from build123d import *

# Parameters (mm, degrees)
BOSS_EXTRUDE1_DEPTH = 25.4
SKETCH2_R           = 2.159
CUT_EXTRUDE1_DEPTH  = 25.4
SKETCH3_R           = 2.159
CUT_EXTRUDE2_DEPTH  = 25.4


with BuildPart() as part:
    # Sketch1 → Boss-Extrude1 (new body)
    with BuildSketch(Plane.XY):
        Polygon((-9.009241013, -10.149737798), (-28.059241013, -10.149737798), (-28.059241013, -6.974737798), (-12.819241013, -6.974737798), (-12.819241013, 5.598262202), (6.738758987, 5.598262202), (6.738758987, -6.974737798), (21.978758987, -6.974737798), (21.978758987, -10.149737798), (2.928758987, -10.149737798), (2.928758987, 1.788262202), (-9.009241013, 1.788262202), align=None)
    extrude(amount=BOSS_EXTRUDE1_DEPTH)

    # Sketch2 → Cut-Extrude1 (cut)
    with BuildSketch(Plane(origin=(0, -6.974737798, 0), x_dir=(1, 0, 0), z_dir=(0, 1, 0))):
        with Locations((14.358758987, -12.7)):
            Circle(SKETCH2_R)
    extrude(amount=-CUT_EXTRUDE1_DEPTH, mode=Mode.SUBTRACT)

    # Sketch3 → Cut-Extrude2 (cut)
    with BuildSketch(Plane(origin=(0, -6.974737798, 0), x_dir=(1, 0, 0), z_dir=(0, 1, 0))):
        with Locations((-20.439241013, -12.7)):
            Circle(SKETCH3_R)
    extrude(amount=-CUT_EXTRUDE2_DEPTH, mode=Mode.SUBTRACT)


solid = part.part
For this review, take the finished solid that the model builds, in its own axes (mm). A direction names the side the tool comes from. Give positions to 0.01 mm unless a question says otherwise; leave off trailing zeros. Order: outer loops, then holes, each group sorted by start corner. A loop starts at its lowest first (then second) coordinate and runs counter-clockwise, first axis right, second up. Notation, with made-up numbers: M -15,6.25 L 41,6.25 A18 cw 41,18.25 Z; hole C 81.5,63.5 d1. An arc over 180 degrees is marked long. Answer in a Markdown table with one row per item. Add a question column.
(1) Consider section A-A on y = -7.75. State the section outline as (x, z) points, and give its area (3 significant figures).
(2) For faces 1 (the face through (2.929, -4, 13)), 2 (the face through (6.739, -1, 13)), 3 (the face through (-21, -6.975, 15)), 4 (the face through (-16, -10.15, 13)), 5 (the face through (16.35, -8.54, 13.53)), list the 3-axis set-ups (+Z, -Z, +X, -X, +Y, -Y) from which the entire face can be reached by the end or side of a thin tool; tool diameter is ignored.
(3) Consider section C-C on y = -4.75. State the section outline as (x, z) points, and give its area (3 significant figures).
(4) For pin 1 (4.5 mm diameter, centred on x = 13.5, z = 15, fed in from +Y); pin 2 (6 mm diameter, centred on x = -2.5, z = 9.5, fed in from -Y); pin 3 (2 mm diameter, centred on y = 0, z = 8, fed in from +X); pin 4 (4 mm diameter, centred on x = -20.44, z = 12.7, fed in from -Y) (3 decimals), all flat-tipped, find the tip position at first contact; note any pin that passes through.
(5) Wall thickness on probe 1 along X at (y, z) = (-9.05, 12.7); probe 2 along X at (y, z) = (-3, 12.25); probe 3 along X at (y, z) = (-9, 22.25): over which ranges is each line inside the solid? List them lowest first. Write a range as [from, to].
(6) Consider section B-B on z = 12.7. State the section outline as (x, y) points, and give its area (3 significant figures).
(7) Consider section D-D on x = 16. State the section outline as (y, z) points.
(8) Mouldability with a two-part tool opening along X and no side actions: class faces 6 (the face through (21.979, -9, 13)), 7 (the face through (-12.819, -1, 13)), 8 (the face through (-9.009, -4, 13)) as +X half, -X half, draft (parallel to the pull), parting line (faces both ways), or undercut.
Evaluation:
| question | item | result |
|---|---|---|
| 1 | outline | M -28.06,0 L -9.01,0 L -9.01,25.4 L -28.06,25.4 Z; M 2.93,0 L 21.98,0 L 21.98,25.4 L 2.93,25.4 Z; hole C -20.44,12.7 d4.32; hole C 14.36,12.7 d4.32 |
| 1 | area | 938 mm^2 |
| 2 | face 1 | +Z, -Z, -Y |
| 2 | face 2 | +Z, -Z, +X, +Y |
| 2 | face 3 | +Z, -Z, -X, +Y |
| 2 | face 4 | +Z, -Z, +X, -X, -Y |
| 2 | face 5 | +Y, -Y |
| 3 | outline | M -12.82,0 L -9.01,0 L -9.01,25.4 L -12.82,25.4 Z; M 2.93,0 L 6.74,0 L 6.74,25.4 L 2.93,25.4 Z |
| 3 | area | 194 mm^2 |
| 4 | pin 1 | stops at y = -6.97 |
| 4 | pin 2 | stops at y = 1.79 |
| 4 | pin 3 | stops at x = 6.74 |
| 4 | pin 4 | passes through |
| 5 | probe 1 | x = [-28.06, -22.6], [-18.28, -9.01], [2.93, 12.2], [16.52, 21.98] |
| 5 | probe 2 | x = [-12.82, -9.01], [2.93, 6.74] |
| 5 | probe 3 | x = [-28.06, -9.01], [2.93, 21.98] |
| 6 | outline | M -28.06,-10.15 L -22.6,-10.15 L -22.6,-6.97 L -28.06,-6.97 Z; M -18.28,-10.15 L -9.01,-10.15 L -9.01,1.79 L 2.93,1.79 L 2.93,-10.15 L 12.2,-10.15 L 12.2,-6.97 L 6.74,-6.97 L 6.74,5.6 L -12.82,5.6 L -12.82,-6.97 L -18.28,-6.97 Z; M 16.52,-10.15 L 21.98,-10.15 L 21.98,-6.97 L 16.52,-6.97 Z |
| 6 | area | 235 mm^2 |
| 7 | outline | M -10.15,0 L -6.97,0 L -6.97,11.3 L -10.15,11.3 Z; M -10.15,14.1 L -6.97,14.1 L -6.97,25.4 L -10.15,25.4 Z |
| 8 | face 6 | +X half |
| 8 | face 7 | -X half |
| 8 | face 8 | undercut |
